Verification items for this drawing (mm, ordinates from the low corner). A direction names the side the tool comes from. Round coordinates to 2 decimals unless told otherwise and drop trailing zeros. Order: outer loops, then holes, each group sorted by start corner. A loop starts at its lowest first (then second) coordinate and runs counter-clockwise, first axis right, second up. Notation, with made-up numbers: (4.5, -18.75) - (11.5, -18.75) arc R26 ccw to (11.5, 9.25) - close; hole circle Ø1 at (74, 32). An arc over 180 degrees is marked (long way). One line per question, with ' | ' between items. Start each with the question number.
Q1. Material ranges on line 1 along X through (y, z) = (8.75, 58); line 2 along Z through (x, y) = (16.5, 8); line 3 along Y through (x, z) = (32, 40), recorded low to high.
Q2. Sectioned sample at B-B, the plane x = 54. Enter the section's corners in (y, z), then the cut area to 3 significant figures.
Q3. Sectioned sample at C-C, the plane y = 8.5. Enter the section's corners in (x, z).
Q4. Tool access check on the marked faces 1 and 2. Record the directions out of +Z, -Z, +X, -X, +Y, -Y that give a thin tool (end or side, any length) a straight path to the whole face; none if there is none.
Q5. Mould release check, pull along Z, two halves, no side actions. Record for the marked faces 3, 4 and 5: +Z half, -Z half, draft (parallel to the pull), parting line (faces both ways), or undercut.
Q6. Sectioned sample at D-D, the plane z = 30. Enter the section's corners in (x, y).
Q7. Gauge pin test, flat ends, axial feed: P1, Ø1.5, axis at y = 18, z = 117, coming from the -X side; P2, Ø4, axis at y = 18, z = 117.5, coming from the +X side; P3, Ø4, axis at x = 96.5, z = 63, coming from the +Y side; P4, Ø1, axis at x = 82, y = 17, coming from the -Z side. Record the tip position at first contact, or that the pin passes through.
Q8. Sectioned sample at A-A, the plane y = 17.75. Enter the section's corners in (x, z), then the cut area to 3 significant figures.
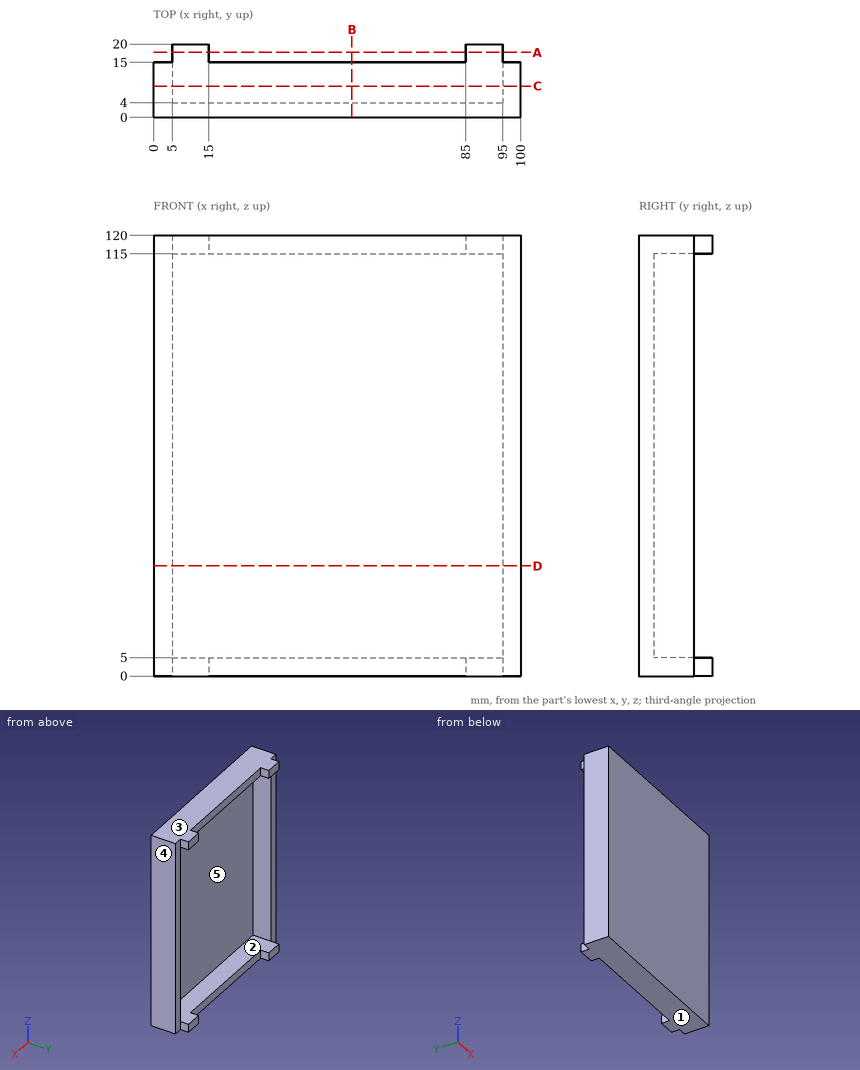
Determined:
1) line 1: x = 0 to 5, 95 to 100 | line 2: z = 0 to 5, 115 to 120 | line 3: y = 0 to 4
2) outline: (0, 0) - (15, 0) - (15, 5) - (4, 5) - (4, 115) - (15, 115) - (15, 120) - (0, 120) - close | area: 590 mm2
3) outline: (0, 0) - (100, 0) - (100, 120) - (0, 120) - close; hole (5, 5) - (95, 5) - (95, 115) - (5, 115) - close
4) face 1: -Z, +X, -X, +Y, -Y | face 2: +Y
5) face 3: +Z half | face 4: draft | face 5: undercut
6) outline: (0, 0) - (100, 0) - (100, 15) - (95, 15) - (95, 4) - (5, 4) - (5, 15) - (0, 15) - close
7) P1: stops at x = 5 | P2: stops at x = 95 | P3: stops at y = 15 | P4: passes through
8) outline: (5, 0) - (15, 0) - (15, 5) - (5, 5) - close; (5, 115) - (15, 115) - (15, 120) - (5, 120) - close; (85, 0) - (95, 0) - (95, 5) - (85, 5) - close; (85, 115) - (95, 115) - (95, 120) - (85, 120) - close | area: 200 mm2
